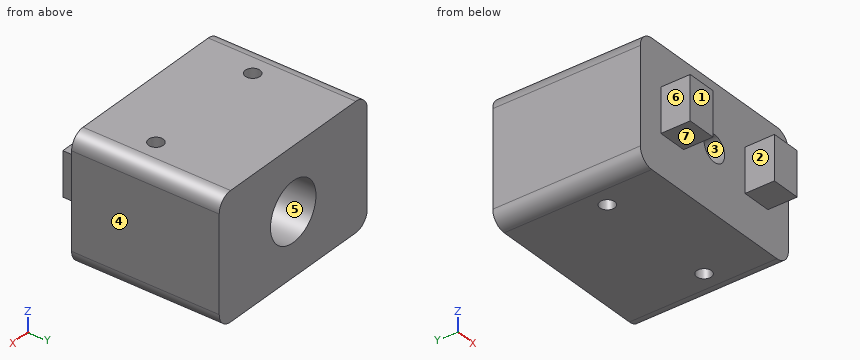
Autodesk Inventor part; units mm, degrees
ref_plane "YZ Plane" through (0, 0, 0) normal (1, 0, 0) x (0, 1, 0)
ref_plane "XZ Plane" through (0, 0, 0) normal (0, 1, 0) x (-1, 0, 0)
ref_plane "XY Plane" through (0, 0, 0) normal (0, 0, 1) x (1, 0, 0)
sketch "Boceto1" plane through (0, 0, 0) normal (0, 1, 0) x (-1, 0, 0)
  line L0 (0, 0) -> (0, -8.5)
  line L1 (0, -8.5) -> (13, -8.5)
  line L2 (13, -8.5) -> (13, 0)
  line L3 (13, 0) -> (0, 0)
  circle A0 centre (6.5, -4.25) radius 0.9
  dimension "d0" = 8.5
  dimension "d1" = 13
  dimension "d2" = 1.8
  dimension "d13" = 4.25
extrude "Extrusión1" add sketch "Boceto1" along normal blind 10.06
sketch "Boceto2" plane through (0, 10.06, 0) normal (0, 1, 0) x (1, 0, 0)
  circle A0 centre (-6.5, 4.25) radius 0.9
  point P0 (0, 0)
hole "Agujero1" at (-6.5, 10.06, -4.25) direction (0, -1, 0) diameter 4 depth 7.06
fillet "Empalme1" radius 1 4 edges at (0, 5.03, 0) (0, 5.03, -8.5) (-13, 5.03, 0) (-13, 5.03, -8.5)
sketch "Boceto3" plane through (0, 0, 0) normal (0, -1, 0) x (1, 0, 0)
  line L0 (-1.8, -5.75) -> (-3.8, -5.75)
  line L1 (-3.8, -5.75) -> (-3.8, -2.75)
  line L2 (-3.8, -2.75) -> (-1.8, -2.75)
  line L3 (-1.8, -2.75) -> (-1.8, -5.75)
  line L4 (0, -1) -> (0, -7.5)
  line L5 (-1, -8.5) -> (-12, -8.5)
  line L6 (-9.2, -5.75) -> (-11.2, -5.75)
  line L7 (-11.2, -5.75) -> (-11.2, -2.75)
  line L8 (-11.2, -2.75) -> (-9.2, -2.75)
  line L9 (-9.2, -2.75) -> (-9.2, -5.75)
  line L10 (-12, 0) -> (-1, 0)
  line L11 (-13, -7.5) -> (-13, -1)
  point P0 (0, 0)
  dimension "d14" = 2
  dimension "d15" = 3
  dimension "d16" = 1.8
  dimension "d17" = 2.75
  dimension "d18" = 2
  dimension "d19" = 3
  dimension "d20" = 2.75
  dimension "d21" = 1.8
extrude "Extrusión2" add sketch "Boceto3" along normal blind 2
sketch "Boceto4" plane through (-12, 0, 0) normal (0, 0, 1) x (1, 0, 0)
  circle A0 centre (1.25, 4) radius 0.5
  circle A1 centre (9.75, 4) radius 0.5
  line L0 (-1, 10.06) -> (-1, 0)
  line L1 (12, 0) -> (12, 10.06)
  line L2 (0, 0) -> (11, 0)
  dimension "d24" = 1
  dimension "d25" = 1
  dimension "d26" = 2.25
  dimension "d27" = 2.25
  dimension "d28" = 4
  dimension "d29" = 4
hole "Agujero2" at (-10.75, 4, 0) at (-2.25, 4, 0) direction (0, 0, -1) diameter 1 end through all
properties part number "Soporte placa 2.0"
The model under review builds one solid part; all positions refer to its coordinate system, in mm. Face numbers are marked on the shaded views. A direction names the side the tool comes from. Coordinates: 2 decimals unless noted, no trailing zeros. Write each loop counter-clockwise with the first axis right and the second up, starting at its lowest first coordinate (ties: lowest second). Pieces come first, ordered by that corner, then holes. Notation, with made-up numbers: (19.25, 36.25) - (38.25, 36.25) arc R18 ccw to (38.25, 63.25) - close; hole circle Ø5 at (85.25, 73.5). An arc over 180 degrees is marked (long way). Answer in a Markdown table with one row per item. Add a question column.
Q1. To check wall thickness, follow line 1 along X through (y, z) = (4, -6.5); line 2 along Z through (x, y) = (-6.5, 1.6); line 3 along X through (y, z) = (0.9, -4.25). State the ranges of each line that lie inside material, in increasing order. Write a range as from..to.
Q2. Consider section A-A on z = -4.25. Give the boundary of the cut face in (x, y).
Q3. For the marked faces 5, 6 and 7, list the 3-axis set-ups (+Z, -Z, +X, -X, +Y, -Y) from which the entire face can be reached by the end or side of a thin tool; tool diameter is ignored.
Q4. Clearance check with flat-ended pins moving along their axes: pin 1 (1.2 mm diameter, centred on x = -7, z = -4.5, fed in from +Y); pin 2 (1 mm diameter, centred on x = -10, y = -1.5, fed in from +Z); pin 3 (1.6 mm diameter, centred on y = -1.5, z = -4.5, fed in from +X). State where each tip first meets the part, or that it passes through.
Q5. Consider section B-B on x = -2.25. Give the boundary of the cut face in (y, z), then the cut area to 3 significant figures.
Q6. Consider section C-C on y = 5.5. Give the boundary of the cut face in (x, z).
Q7. Consider section D-D on z = -7. Give the boundary of the cut face in (x, y).
Q8. Draft analysis for pull direction X (two halves, no side actions). For the marked faces 1, 2, 3 and 4, state which applies: +X half, -X half, draft (parallel to the pull), parting line (faces both ways), or undercut.
Answers below:
| question | item | result |
|---|---|---|
| 1 | line 1 | -13..-11.25, -10.25..-2.75, -1.75..0 |
| 1 | line 2 | -8.5..-5.15, -3.35..0 |
| 1 | line 3 | -13..-7.4, -5.6..0 |
| 2 | outline | (-13, 0) - (-11.2, 0) - (-11.2, -2) - (-9.2, -2) - (-9.2, 0) - (-7.4, 0) - (-7.4, 3) - (-8.5, 3) - (-8.5, 10.06) - (-13, 10.06) - close; (-5.6, 0) - (-3.8, 0) - (-3.8, -2) - (-1.8, -2) - (-1.8, 0) - (0, 0) - (0, 10.06) - (-4.5, 10.06) - (-4.5, 3) - (-5.6, 3) - close; hole circle Ø1 at (-10.75, 4); hole circle Ø1 at (-2.25, 4) |
| 3 | face 5 | +Y |
| 3 | face 6 | +Z, -Z, -X, -Y |
| 3 | face 7 | -Z, +X, -X, -Y |
| 4 | pin 1 | y = 3 |
| 4 | pin 2 | z = -2.75 |
| 4 | pin 3 | x = -1.8 |
| 5 | outline | (-2, -5.75) - (0, -5.75) - (0, -8.5) - (3.5, -8.5) - (3.5, 0) - (0, 0) - (0, -2.75) - (-2, -2.75) - close; (4.5, -8.5) - (10.06, -8.5) - (10.06, 0) - (4.5, 0) - close |
| 5 | area | 83.0 mm² |
| 6 | outline | (-13, -7.5) arc R1 ccw to (-12, -8.5) - (-1, -8.5) arc R1 ccw to (0, -7.5) - (0, -1) arc R1 ccw to (-1, 0) - (-12, 0) arc R1 ccw to (-13, -1) - close; hole circle Ø4 at (-6.5, -4.25) |
| 7 | outline | (-13, 0) - (0, 0) - (0, 10.06) - (-13, 10.06) - close; hole circle Ø1 at (-10.75, 4); hole circle Ø1 at (-2.25, 4) |
| 8 | face 1 | draft |
| 8 | face 2 | undercut |
| 8 | face 3 | undercut |
| 8 | face 4 | +X half |
